```python
from build123d import *

# Parameters (mm, degrees)
SKETCH2_W           = 112.00010125
SKETCH2_H           = 190.5995575
SKETCH2_R           = 2.1
SKETCH2_R_2         = 1.85
BOSS_EXTRUDE1_DEPTH = 1.2
SKETCH5_W           = 2
SKETCH5_H           = 37.6
SKETCH5_H_2         = 0.6
CUT_EXTRUDE2_DEPTH  = 247.246128205
CUT_EXTRUDE1_DEPTH  = 247.246128205
SKETCH9_W           = 14
SKETCH9_H           = 3.4
SKETCH9_W_2         = 8.5
BOSS_EXTRUDE5_DEPTH = 1.2
FILLET1_R           = 1
CUT_EXTRUDE4_REACH  = 248.246
SKETCH10_W          = 8.2
SKETCH10_H          = 0.7
SKETCH11_R          = 2.25
CUT_EXTRUDE5_DEPTH  = 247.246128205
BOSS_EXTRUDE6_DEPTH = 1.2
SKETCH13_R          = 1.635773904
CUT_EXTRUDE6_DEPTH  = 248.202612706
SKETCH14_W          = 1.2
SKETCH14_H          = 152.3995575
BOSS_EXTRUDE7_DEPTH = 32
BOSS_EXTRUDE8_DEPTH = 1.2
BOSS_EXTRUDE9_DEPTH = 1.2
CUT_EXTRUDE7_REACH  = 254.685
FILLET2_R           = 1


with BuildPart() as part:
    # Sketch2 → Boss-Extrude1 (new body)
    with BuildSketch(Plane.XY):
        with Locations((50.167238625, 126.88082875)):
            Rectangle(SKETCH2_W, SKETCH2_H)
        with Locations((8.16763175, 151.180160625)):
            Circle(SKETCH2_R, mode=Mode.SUBTRACT)
        with Locations((100.1668405, 151.180160625)):
            Circle(SKETCH2_R_2, mode=Mode.SUBTRACT)
        with Locations((100.1668405, 36.181495)):
            Circle(SKETCH2_R_2, mode=Mode.SUBTRACT)
        with Locations((8.16763175, 36.181495)):
            Circle(SKETCH2_R, mode=Mode.SUBTRACT)
    extrude(amount=BOSS_EXTRUDE1_DEPTH)

    # Sketch5 → Cut-Extrude2 (cut, through all)
    with BuildSketch(Plane.XY.offset(1.2)):
        Polygon((-3.832812, 185.1806075), (6.667188, 185.1806075), (6.667188, 222.1806075), (-5.832812, 222.1806075), (-5.832812, 185.1806075), (-5.832812, 184.5806075), (-3.832812, 184.5806075), align=None)
        with Locations((105.16728925, 203.3806075)):
            Rectangle(SKETCH5_W, SKETCH5_H)
        with Locations((-4.832812, 31.88105)):
            Rectangle(SKETCH5_W, SKETCH5_H_2)
        with Locations((105.16728925, 31.88105)):
            Rectangle(SKETCH5_W, SKETCH5_H_2)
    extrude(amount=-CUT_EXTRUDE2_DEPTH, mode=Mode.SUBTRACT)

    # Sketch4 → Cut-Extrude1 (cut, through all)
    with BuildSketch(Plane.XY.offset(1.2)):
        with BuildLine():
            Line((55.16728925, 218.1806075), (98.16728925, 218.1806075))
            ThreePointArc((98.16728925, 218.1806075), (99.581502812, 217.594821062), (100.16728925, 216.1806075))
            Line((100.16728925, 216.1806075), (100.16728925, 192.1806075))
            ThreePointArc((100.16728925, 192.1806075), (99.581502812, 190.766393938), (98.16728925, 190.1806075))
            Line((98.16728925, 190.1806075), (55.16728925, 190.1806075))
            ThreePointArc((55.16728925, 190.1806075), (53.753075688, 190.766393938), (53.16728925, 192.1806075))
            Line((53.16728925, 192.1806075), (53.16728925, 216.1806075))
            ThreePointArc((53.16728925, 216.1806075), (53.753075688, 217.594821062), (55.16728925, 218.1806075))
        make_face()
    extrude(amount=-CUT_EXTRUDE1_DEPTH, mode=Mode.SUBTRACT)

    # Sketch9 → Boss-Extrude5 (add)
    with BuildSketch(Plane.XY.offset(1.2)):
        with Locations((5.167188, 29.88105)):
            Rectangle(SKETCH9_W, SKETCH9_H)
        with Locations((95.16728925, 29.88105)):
            Rectangle(SKETCH9_W, SKETCH9_H)
        with Locations((50.167238625, 29.88105)):
            Rectangle(SKETCH9_W, SKETCH9_H)
        with Locations((2.417188, 186.8806075)):
            Rectangle(SKETCH9_W_2, SKETCH9_H)
    extrude(amount=-BOSS_EXTRUDE5_DEPTH)

    # Fillet1
    fillet1_edges = [part.edges().sort_by_distance(p)[0] for p in [
        (102.16728925, 28.18105, 0.6),
        (88.16728925, 28.18105, 0.6),
        (57.167238625, 28.18105, 0.6),
        (43.167238625, 28.18105, 0.6),
        (12.167188, 28.18105, 0.6),
        (-1.832812, 28.18105, 0.6),
        (-1.832812, 188.5806075, 0.6),
    ]]
    fillet(fillet1_edges, radius=FILLET1_R)

    # Sketch10 → Cut-Extrude4 (cut, up to next)
    with BuildSketch(Plane.XY.offset(1.2), mode=Mode.PRIVATE) as cut_extrude4_sk1:
        with Locations((95.16728925, 31.93105)):
            Rectangle(SKETCH10_W, SKETCH10_H)
    cut_extrude4_tool1 = extrude(cut_extrude4_sk1.sketch, amount=-CUT_EXTRUDE4_REACH, mode=Mode.PRIVATE) & part.part
    # Sketch10 → Cut-Extrude4 (cut, up to next)
    with BuildSketch(Plane.XY.offset(1.2), mode=Mode.PRIVATE) as cut_extrude4_sk2:
        with Locations((50.167238625, 31.93105)):
            Rectangle(SKETCH10_W, SKETCH10_H)
    cut_extrude4_tool2 = extrude(cut_extrude4_sk2.sketch, amount=-CUT_EXTRUDE4_REACH, mode=Mode.PRIVATE) & part.part
    # Sketch10 → Cut-Extrude4 (cut, up to next)
    with BuildSketch(Plane.XY.offset(1.2), mode=Mode.PRIVATE) as cut_extrude4_sk3:
        with Locations((5.167188, 31.93105)):
            Rectangle(SKETCH10_W, SKETCH10_H)
    cut_extrude4_tool3 = extrude(cut_extrude4_sk3.sketch, amount=-CUT_EXTRUDE4_REACH, mode=Mode.PRIVATE) & part.part
    # Sketch10 → Cut-Extrude4 (cut, up to next)
    with BuildSketch(Plane.XY.offset(1.2), mode=Mode.PRIVATE) as cut_extrude4_sk4:
        with Locations((50.167238625, 184.8306075)):
            Rectangle(SKETCH10_W, SKETCH10_H)
    cut_extrude4_tool4 = extrude(cut_extrude4_sk4.sketch, amount=-CUT_EXTRUDE4_REACH, mode=Mode.PRIVATE) & part.part
    # Sketch10 → Cut-Extrude4 (cut, up to next)
    with BuildSketch(Plane.XY.offset(1.2), mode=Mode.PRIVATE) as cut_extrude4_sk5:
        with Locations((95.16728925, 184.8306075)):
            Rectangle(SKETCH10_W, SKETCH10_H)
    cut_extrude4_tool5 = extrude(cut_extrude4_sk5.sketch, amount=-CUT_EXTRUDE4_REACH, mode=Mode.PRIVATE) & part.part
    # Sketch10 → Cut-Extrude4 (cut, up to next)
    with BuildSketch(Plane.XY.offset(1.2), mode=Mode.PRIVATE) as cut_extrude4_sk6:
        with Locations((5.167188, 184.8306075)):
            Rectangle(SKETCH10_W, SKETCH10_H)
    cut_extrude4_tool6 = extrude(cut_extrude4_sk6.sketch, amount=-CUT_EXTRUDE4_REACH, mode=Mode.PRIVATE) & part.part
    add(cut_extrude4_tool1.solids().sort_by_distance((95.167289, 31.93105, 1.2))[0], mode=Mode.SUBTRACT)
    add(cut_extrude4_tool2.solids().sort_by_distance((50.167239, 31.93105, 1.2))[0], mode=Mode.SUBTRACT)
    add(cut_extrude4_tool3.solids().sort_by_distance((5.167188, 31.93105, 1.2))[0], mode=Mode.SUBTRACT)
    add(cut_extrude4_tool4.solids().sort_by_distance((50.167239, 184.830607, 1.2))[0], mode=Mode.SUBTRACT)
    add(cut_extrude4_tool5.solids().sort_by_distance((95.167289, 184.830607, 1.2))[0], mode=Mode.SUBTRACT)
    add(cut_extrude4_tool6.solids().sort_by_distance((5.167188, 184.830607, 1.2))[0], mode=Mode.SUBTRACT)

    # Sketch11 → Cut-Extrude5 (cut, through all)
    with BuildSketch(Plane.XY.offset(1.2)):
        with Locations((61.367697375, 160.67994375)):
            Circle(SKETCH11_R)
        with Locations((13.067697375, 172.47994375)):
            Circle(SKETCH11_R)
        with BuildLine():
            Line((71.867697375, 175.27994375), (71.867697375, 170.27994375))
            ThreePointArc((71.867697375, 170.27994375), (69.367697375, 167.77994375), (66.867697375, 170.27994375))
            Line((66.867697375, 170.27994375), (66.867697375, 175.27994375))
            ThreePointArc((66.867697375, 175.27994375), (69.367697375, 177.77994375), (71.867697375, 175.27994375))
        make_face()
    extrude(amount=-CUT_EXTRUDE5_DEPTH, mode=Mode.SUBTRACT)

    # Sketch12 → Boss-Extrude6 (add)
    with BuildSketch(Plane.XY.offset(1.2)):
        with BuildLine():
            Line((104.16728925, 222.1806075), (104.16728925, 213.7806075))
            ThreePointArc((104.16728925, 213.7806075), (108.36728925, 217.9806075), (104.16728925, 222.1806075))
        make_face()
    extrude(amount=-BOSS_EXTRUDE6_DEPTH)

    # Sketch13 → Cut-Extrude6 (cut, through all)
    with BuildSketch(Plane.XY.offset(1.2)):
        with Locations((104.16728925, 217.9806075)):
            Circle(SKETCH13_R)
        with Locations((47.16728925, 217.9806075)):
            Circle(SKETCH13_R)
        with Locations((10.667188, 217.9806075)):
            Circle(SKETCH13_R)
    extrude(amount=-CUT_EXTRUDE6_DEPTH, mode=Mode.SUBTRACT)

    # Sketch14 → Boss-Extrude7 (add)
    with BuildSketch(Plane(origin=(0, 0, 0), x_dir=(-1, 0, 0), z_dir=(0, 0, -1))):
        with Locations((5.232812, 108.38082875)):
            Rectangle(SKETCH14_W, SKETCH14_H)
    extrude(amount=BOSS_EXTRUDE7_DEPTH)

    # Sketch16 → Boss-Extrude8 (add)
    with BuildSketch(Plane.ZY.offset(5.832812)):
        with BuildLine():
            Line((-32, 32.18105), (-4, 32.18105))
            ThreePointArc((-4, 32.18105), (-6.121320344, 31.302370344), (-7, 29.18105))
            Line((-7, 29.18105), (-7, 18.18105))
            Line((-7, 18.18105), (-32, 18.18105))
            Line((-32, 18.18105), (-32, 32.18105))
        make_face()
    extrude(amount=-BOSS_EXTRUDE8_DEPTH)

    # Sketch17 → Boss-Extrude9 (add)
    with BuildSketch(Plane.ZY.offset(5.832812)):
        with BuildLine():
            Line((-32, 184.5806075), (-38, 184.5806075))
            Line((-38, 184.5806075), (-38, 168.5806075))
            Line((-38, 168.5806075), (-35, 168.5806075))
            ThreePointArc((-35, 168.5806075), (-32.878679656, 167.701927844), (-32, 165.5806075))
            Line((-32, 165.5806075), (-32, 184.5806075))
        make_face()
    extrude(amount=-BOSS_EXTRUDE9_DEPTH)

    # Sketch15 → Cut-Extrude7 (cut, up to next)
    with BuildSketch(Plane.ZY.offset(5.832812), mode=Mode.PRIVATE) as cut_extrude7_sk1:
        with BuildLine():
            Line((-46.8, 177.7806075), (-34.8, 177.7806075))
            ThreePointArc((-34.8, 177.7806075), (-33.2, 176.1806075), (-34.8, 174.5806075))
            Line((-34.8, 174.5806075), (-46.8, 174.5806075))
            ThreePointArc((-46.8, 174.5806075), (-48.4, 176.1806075), (-46.8, 177.7806075))
        make_face()
    cut_extrude7_tool1 = extrude(cut_extrude7_sk1.sketch, amount=-CUT_EXTRUDE7_REACH, mode=Mode.PRIVATE) & part.part
    # Sketch15 → Cut-Extrude7 (cut, up to next)
    with BuildSketch(Plane.ZY.offset(5.832812), mode=Mode.PRIVATE) as cut_extrude7_sk2:
        with BuildLine():
            Line((-26.1, 21.18105), (-26.1, 18.18105))
            Line((-26.1, 18.18105), (-22.9, 18.18105))
            Line((-22.9, 18.18105), (-22.9, 21.18105))
            ThreePointArc((-22.9, 21.18105), (-24.5, 22.78105), (-26.1, 21.18105))
        make_face()
    cut_extrude7_tool2 = extrude(cut_extrude7_sk2.sketch, amount=-CUT_EXTRUDE7_REACH, mode=Mode.PRIVATE) & part.part
    add(cut_extrude7_tool1.solids().sort_by_distance((-5.832812, 176.180608, -40.8))[0], mode=Mode.SUBTRACT)
    add(cut_extrude7_tool2.solids().sort_by_distance((-5.832812, 20.324349, -24.5))[0], mode=Mode.SUBTRACT)

    # Fillet2
    fillet2_edges = [part.edges().sort_by_distance(p)[0] for p in [
        (6.667188, 222.1806075, 0.6),
        (-5.232812, 18.18105, -32),
        (-5.232812, 18.18105, -7),
        (-5.232812, 168.5806075, -38),
        (-5.232812, 184.5806075, -38),
    ]]
    fillet(fillet2_edges, radius=FILLET2_R)


solid = part.part
```
Could you check a few things on this model? Use its own coordinates, in mm. A direction names the side the tool comes from. Coordinates: 2 decimals unless noted, no trailing zeros. Order: outer loops, then holes, each group sorted by start corner. A loop starts at its lowest first (then second) coordinate and runs counter-clockwise, first axis right, second up. Notation, with made-up numbers: M 32.5,50.25 L 80.5,50.25 A20 cw 80.5,75.25 Z; hole C 22.5,-4.5 d4. An arc over 180 degrees is marked long. Use a Markdown table: item, result. Add a question column.
Q1. I want a section at D-D on z = -19.5. List the corners of the cut face in (x, y) for me, then the cut area to 3 significant figures.
Q2. I'm going to push flat-ended pins straight in: pin 1 (1 mm diameter, centred on x = -5.5, y = 24.5, fed in from +Z); pin 2 (10 mm diameter, centred on x = 18, y = 164, fed in from -Z); pin 3 (1 mm diameter, centred on x = 51, z = 0.5, fed in from -Y); pin 4 (2 mm diameter, centred on x = 47.17, y = 217.98, fed in from +Z). Where does each tip first touch, or does it pass through?
Q3. If I drill on L1, parallel to Z at x = 96, y = 30.5; L2, parallel to X at y = 173, z = -11, over which ranges is the centre line in solid material (lowest first)?
Q4. I want a section at A-A on x = 79.5. List the corners of the cut face in (y, z) for me.
Q5. We'd pull the mould along X, two halves only. Please class faces 3 (the cylindrical face through (9.1, 34.3, 0.6)), 4 (the flat face through (-5.833, 103, -19)), 5 (the cylindrical face through (108.366, 217.888, 0.608)): pulls with the +X half, pulls with the -X half, needs draft (parallel to the pull), parting line crosses it, or undercut.
Q6. Which directions (+Z, -Z, +X, -X, +Y, -Y) give clear straight access to the entire face, cutting with the end or side of a thin tool? Please do faces 1 (the flat face through (51, 127, 0)), 2 (the cylindrical face through (12.77, 174.71, 0.61)).
Q7. I want a section at B-B on x = 94. List the corners of the cut face in (y, z) for me.
Q8. I want a section at C-C on y = 85. List the corners of the cut face in (x, z) for me, then the cut area to 3 significant figures.
Checked values:
| question | item | result |
|---|---|---|
| 1 | outline | M -5.83,18.18 L -4.63,18.18 L -4.63,184.58 L -5.83,184.58 Z |
| 1 | area | 200 mm² |
| 2 | pin 1 | z = -7 |
| 2 | pin 2 | z = 0 |
| 2 | pin 3 | y = 28.18 |
| 2 | pin 4 | through |
| 3 | L1 | 0 to 1.2 |
| 3 | L2 | -5.83 to -4.63 |
| 4 | outline | M 31.58,0 L 190.18,0 L 190.18,1.2 L 31.58,1.2 Z; M 218.18,0 L 222.18,0 L 222.18,1.2 L 218.18,1.2 Z |
| 5 | face 3 | undercut |
| 5 | face 4 | pulls with the -X half |
| 5 | face 5 | pulls with the +X half |
| 6 | face 1 | -Z, +X, +Y, -Y |
| 6 | face 2 | +Z, -Z |
| 7 | outline | M 28.18,0 L 31.58,0 L 31.58,1.2 L 28.18,1.2 Z; M 32.28,0 L 184.48,0 L 184.48,1.2 L 32.28,1.2 Z; M 185.18,0 L 190.18,0 L 190.18,1.2 L 185.18,1.2 Z; M 218.18,0 L 222.18,0 L 222.18,1.2 L 218.18,1.2 Z |
| 8 | outline | M -5.83,-32 L -4.63,-32 L -4.63,0 L 106.17,0 L 106.17,1.2 L -5.83,1.2 Z |
| 8 | area | 173 mm² |
